from build123d import *

# Parameters (mm, degrees)
SKETCH1_W           = 300
SKETCH1_H           = 200
BOSS_EXTRUDE1_DEPTH = 5
SKETCH3_W           = 20
SKETCH3_H           = 20
SKETCH3_H_2         = 40
CUT_EXTRUDE1_DEPTH  = 5
SKETCH4_W           = 20
SKETCH4_H           = 40
CUT_EXTRUDE2_DEPTH  = 10


with BuildPart() as part:
    # Sketch1 → Boss-Extrude1 (new body)
    with BuildSketch(Plane.XY):
        Rectangle(SKETCH1_W, SKETCH1_H)
    extrude(amount=BOSS_EXTRUDE1_DEPTH)

    # Sketch3 → Cut-Extrude1 (cut)
    with BuildSketch(Plane.XY.offset(5)):
        with Locations((-140, -90)):
            Rectangle(SKETCH3_W, SKETCH3_H)
        with Locations((-140, 80)):
            Rectangle(SKETCH3_W, SKETCH3_H_2)
        with Locations((140, 80)):
            Rectangle(SKETCH3_W, SKETCH3_H_2)
        with Locations((140, -90)):
            Rectangle(SKETCH3_W, SKETCH3_H)
    extrude(amount=-CUT_EXTRUDE1_DEPTH, mode=Mode.SUBTRACT)

    # Sketch4 → Cut-Extrude2 (cut)
    with BuildSketch(Plane(origin=(0, 0, 0), x_dir=(-1, 0, 0), z_dir=(0, 0, -1))):
        with Locations((-140, -80)):
            Rectangle(SKETCH4_W, SKETCH4_H)
        with Locations((140, -80)):
            Rectangle(SKETCH4_W, SKETCH4_H)
    extrude(amount=-CUT_EXTRUDE2_DEPTH, mode=Mode.SUBTRACT)


solid = part.part
Read the model definition and answer for the solid it produces. Units are mm, in the model's axes. Round coordinates to 2 decimals unless told otherwise and drop trailing zeros. Order: outer loops, then holes, each group sorted by start corner. A loop starts at its lowest first (then second) coordinate and runs counter-clockwise, first axis right, second up.
1) The part is cut by section B-B on y = 76. Write down the section's boundary in (x, z).
2) The part is cut by section A-A on z = 2.7. Write down the section's boundary in (x, y), plus the area to 3 significant figures.
3) A straight line is drawn through the part: L1, parallel to X at y = -78, z = 2.3. Find the intervals that lie inside material, in ascending order.
4) Flat-ended cylindrical pins translate along their axes: pin 1 (2.5 mm diameter, centred on y = 78, z = 3.5, fed in from +X); pin 2 (3 mm diameter, centred on x = -13.5, y = -66, fed in from -Z); pin 3 (2.5 mm diameter, centred on x = -136.5, z = 3.5, fed in from -Y); pin 4 (2.5 mm diameter, centred on y = 79, z = 2.5, fed in from -X). Find the tip coordinate at first contact, or state that the pin passes through.
Resolved:
1. outline: (-130, 0) - (130, 0) - (130, 5) - (-130, 5) - close
2. outline: (-150, -60) - (-130, -60) - (-130, -100) - (130, -100) - (130, -60) - (150, -60) - (150, 60) - (130, 60) - (130, 100) - (-130, 100) - (-130, 60) - (-150, 60) - close
2. area: 56,800 mm2
3. L1: x = -130 to 130
4. pin 1: stops at x = 130
4. pin 2: stops at z = 0
4. pin 3: stops at y = -60
4. pin 4: stops at x = -130
